```python
from build123d import *

# Parameters (mm, degrees)
SKETCH_1_W          = 70
SKETCH_1_H          = 75
EXTRUDE_1_DEPTH     = 4
EXTRUDE_2_DEPTH     = 250
CUT_EXTRUDE_1_DEPTH = 263.309454652
SKETCH_4_R          = 14
SKETCH_4_R_2        = 10
EXTRUDE_3_DEPTH     = 40


with BuildPart() as part:
    # 草图1 → 凸台-拉伸1 (new body)
    with BuildSketch(Plane.XY):
        Rectangle(SKETCH_1_W, SKETCH_1_H)
    extrude(amount=EXTRUDE_1_DEPTH)

    # 草图2 → 凸台-拉伸2 (add)
    with BuildSketch(Plane(origin=(0, 0, 0), x_dir=(-1, 0, 0), z_dir=(0, 0, -1))):
        Polygon((35, 37.5), (35, -37.5), (-35, -37.5), (-35, 37.5), (-31, 37.5), (-31, -33.5), (31, -33.5), (31, 37.5), align=None)
    extrude(amount=EXTRUDE_2_DEPTH)

    # 草图3 → 切除-拉伸1 (cut, through all)
    with BuildSketch(Plane.ZY.offset(35)):
        Polygon((4, 37.5), (-250, 37.5), (-250, 12.5), align=None)
    extrude(amount=-CUT_EXTRUDE_1_DEPTH, mode=Mode.SUBTRACT)

    # 草图4 → 凸台-拉伸3 (add)
    with BuildSketch(Plane.XY.offset(4)):
        with Locations(Location((0, 0, 0), (0, 0, 180))):
            Circle(SKETCH_4_R)
        Circle(SKETCH_4_R_2, mode=Mode.SUBTRACT)
    extrude(amount=EXTRUDE_3_DEPTH)


solid = part.part
```
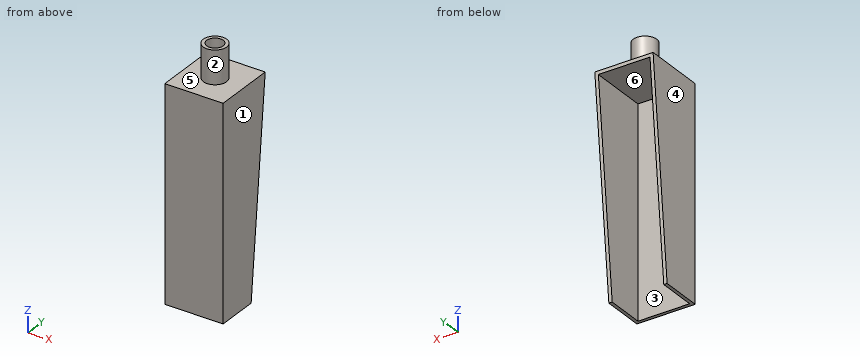
Work out the finished part from the listing and answer in its coordinate system (mm). Face numbers are marked on the shaded views. A direction names the side the tool comes from. Round coordinates to 2 decimals unless told otherwise and drop trailing zeros. Order: outer loops, then holes, each group sorted by start corner. A loop starts at its lowest first (then second) coordinate and runs counter-clockwise, first axis right, second up.
Q1. Given pin 1 Ø6 at (x, y) = (-3, 2) entering from -Z; pin 2 Ø6 at (x, y) = (-3.5, 2.5) entering from +Z; pin 3 Ø1.5 at (x, z) = (-1.5, -124.5) entering from +Y, each flat-ended and moving along its own axis, determine where each tip first touches the part or whether it passes through.
Solution:
pin 1: stops at z = 0
pin 2: stops at z = 4
pin 3: stops at y = -33.5
Q2. A tool of negligible diameter and unlimited length cuts with its end or side. For the marked faces 4, 5 and 6, from which of +Z, -Z, +X, -X, +Y, -Y can it reach the whole face along a straight path? Write none if from no direction.
Solution:
face 4: +Z, -Z, -X, +Y, -Y
face 5: +Z
face 6: -Z, +Y
Q3. A cutting plane is placed at B-B, the plane y = 0. Determine the outline of the cut face in (x, z), then the cut area to 3 significant figures.
Solution:
outline: (-35, -250) - (-31, -250) - (-31, 0) - (31, 0) - (31, -250) - (35, -250) - (35, 4) - (14, 4) - (14, 44) - (10, 44) - (10, 4) - (-10, 4) - (-10, 44) - (-14, 44) - (-14, 4) - (-35, 4) - close
area: 2,600 mm2
Q4. Find the intervals of material crossed by line 1 along Y through (x, z) = (0, 15); line 2 along X through (y, z) = (9, -32); line 3 along Y through (x, z) = (-11, -154.5), in increasing order.
Solution:
line 1: y = -14 to -10, 10 to 14
line 2: x = -35 to -31, 31 to 35
line 3: y = -37.5 to -33.5
Q5. The mould has two halves that part along X. Classify the marked faces 1, 2 and 3: pulls with the +X half, pulls with the -X half, needs draft (parallel to the pull), parting line crosses it, or undercut.
Solution:
face 1: pulls with the +X half
face 2: parting line crosses it
face 3: undercut
Q6. A cutting plane is placed at D-D, the plane z = -197.5. Determine the outline of the cut face in (x, y), then the cut area to 3 significant figures.
Solution:
outline: (-35, -37.5) - (35, -37.5) - (35, 17.67) - (31, 17.67) - (31, -33.5) - (-31, -33.5) - (-31, 17.67) - (-35, 17.67) - close
area: 689 mm2
Q7. A cutting plane is placed at A-A, the plane x = 0. Determine the outline of the cut face in (y, z), then the cut area to 3 significant figures.
Solution:
outline: (-37.5, -250) - (-33.5, -250) - (-33.5, 0) - (37.11, 0) - (37.5, 4) - (14, 4) - (14, 44) - (10, 44) - (10, 4) - (-10, 4) - (-10, 44) - (-14, 44) - (-14, 4) - (-37.5, 4) - close
area: 1,620 mm2
Q8. A cutting plane is placed at C-C, the plane z = 7. Determine the outline of the cut face in (x, y).
Solution:
outline: circle Ø28 at (0, 0); hole circle Ø20 at (0, 0)
